```python
from build123d import *

# Parameters (mm, degrees)
BOSS_EXTRUDE1_DEPTH      = 15.875
S_0_348_DIAMETER_HOLE1_D = 8.8392
S_0_348_DIAMETER_HOLE2_D = 8.8392
FILLET1_R                = 6.35


with BuildPart() as part:
    # Sketch1 → Boss-Extrude1 (new, symmetric)
    with BuildSketch(Plane.XY):
        with BuildLine():
            Line((0, 0), (76.2, 0))
            ThreePointArc((76.2, 0), (74.340128061, 4.490128061), (69.85, 6.35))
            Line((69.85, 6.35), (6.35, 6.35))
            Line((6.35, 6.35), (6.35, 69.85))
            ThreePointArc((6.35, 69.85), (4.490128061, 74.340128061), (0, 76.2))
            Line((0, 76.2), (0, 0))
        make_face()
    extrude(amount=BOSS_EXTRUDE1_DEPTH, both=True)

    # S (0.348) Diameter Hole1 (through all)
    with Locations(Plane(origin=(6.35, 0, 0), x_dir=(0, 0, -1), z_dir=(1, 0, 0))):
        with Locations((0, 57.15), (0, 19.05)):
            Hole(S_0_348_DIAMETER_HOLE1_D / 2)

    # S (0.348) Diameter Hole2 (through all)
    with Locations(Plane(origin=(0, 6.35, 0), x_dir=(-1, 0, 0), z_dir=(0, 1, 0))):
        with Locations((-19.05, 0), (-57.15, 0)):
            Hole(S_0_348_DIAMETER_HOLE2_D / 2)

    # Fillet1
    fillet1_edges = [part.edges().sort_by_distance(p)[0] for p in [
        (6.35, 6.35, 0),
    ]]
    fillet(fillet1_edges, radius=FILLET1_R)


solid = part.part
```
The model under review builds one solid part; all positions refer to its coordinate system, in mm. A direction names the side the tool comes from. Round coordinates to 2 decimals unless told otherwise and drop trailing zeros. Loops run counter-clockwise (first coordinate to the right, second up) from the corner with the lowest first, then second, coordinate; pieces in that order, holes last.
1) Consider section D-D on z = -12.5. State the section outline as (x, y) points, then the cut area to 3 significant figures.
Values follow:
outline: (0, 0) - (76.2, 0) arc R6.35 ccw to (69.85, 6.35) - (12.7, 6.35) arc R6.35 cw to (6.35, 12.7) - (6.35, 69.85) arc R6.35 ccw to (0, 76.2) - close
area: 919 mm2
2) Tool access review of faces 4 (the face through (42, 6.35, 0)), 5 (the face through (4, 21, -15.875)): name each direction out of +Z, -Z, +X, -X, +Y, -Y from which nothing blocks a thin tool from reaching the whole face with its end or side.
Values follow:
face 4: +Z, -Z, +X, +Y
face 5: -Z, +X, -X, +Y, -Y
3) Consider section A-A on z = 0. State the section outline as (x, y) points.
Values follow:
outline: (0, 0) - (14.63, 0) - (14.63, 6.35) - (12.7, 6.35) arc R6.35 cw to (6.35, 12.7) - (6.35, 14.63) - (0, 14.63) - close; (0, 23.47) - (6.35, 23.47) - (6.35, 52.73) - (0, 52.73) - close; (0, 61.57) - (6.35, 61.57) - (6.35, 69.85) arc R6.35 ccw to (0, 76.2) - close; (23.47, 0) - (52.73, 0) - (52.73, 6.35) - (23.47, 6.35) - close; (61.57, 0) - (76.2, 0) arc R6.35 ccw to (69.85, 6.35) - (61.57, 6.35) - close
4) Wall thickness on line 1 along Z through (x, y) = (19.05, 2.75) (3 decimals); line 2 along Y through (x, z) = (1.75, 0); line 3 along X through (y, z) = (53, 13): over which ranges is each line inside the solid? List them lowest first.
Values follow:
line 1: z = -15.875 to -4.42, 4.42 to 15.875
line 2: y = 0 to 14.63, 23.47 to 52.73, 61.57 to 75.95
line 3: x = 0 to 6.35
5) Consider section B-B on x = 57.15. State the section outline as (y, z) points (3 decimals), then the cut area to 3 significant figures.
Values follow:
outline: (0, -15.875) - (6.35, -15.875) - (6.35, -4.42) - (0, -4.42) - close; (0, 4.42) - (6.35, 4.42) - (6.35, 15.875) - (0, 15.875) - close
area: 145 mm2
6) The part is to be moulded in two halves that separate along X. For faces 1 (the face through (3.13, 61.53, -0.58)), 2 (the face through (23.266, 3.131, 1.328)), 3 (the face through (6.35, 41, 0)), say which applies: pulls with the +X half, pulls with the -X half, needs draft (parallel to the pull), parting line crosses it, or undercut.
Values follow:
face 1: needs draft
face 2: undercut
face 3: pulls with the +X half
7) Clearance check with flat-ended pins moving along their axes: P1, Ø14, axis at x = 57.15, z = 0, coming from the +Y side; P2, Ø10, axis at y = 35, z = -8.5, coming from the +X side. State where each tip first meets the part, or that it passes through.
Values follow:
P1: stops at y = 6.35
P2: stops at x = 6.35
